from build123d import *

# Parameters (mm, degrees)
F0_R     = 5
F1_DEPTH = 15
F3_DEPTH = 12
F4_SIZE  = 0.3


with BuildPart() as f1:
    # F0 (on Top) → F1 (new body)
    with BuildSketch(Plane.XY):
        Circle(F0_R)
    extrude(amount=F1_DEPTH)

    # F2 (on face) → F3 (cut)
    with BuildSketch(Plane.XY.offset(15)):
        with BuildLine():
            Line((2.097618, 2.35), (-2.097618, 2.35))
            ThreePointArc((-2.097618, 2.35), (0, -3.15), (2.097618, 2.35))
        make_face()
    extrude(amount=-F3_DEPTH, mode=Mode.SUBTRACT)

    # F4
    f4_edges = [f1.edges().sort_by_distance(p)[0] for p in [
        (-5, 0, 0),
    ]]
    chamfer(f4_edges, length=F4_SIZE)


solid = f1.part
Model file for the job. Use its own axes, mm. A direction names the side the tool comes from. Round coordinates to 2 decimals unless told otherwise and drop trailing zeros. Loops run counter-clockwise (first coordinate to the right, second up) from the corner with the lowest first, then second, coordinate; pieces in that order, holes last.
1. Wall check: probe 1 along Y at (x, z) = (0, 10); probe 2 along Z at (x, y) = (1.5, -2); probe 3 along Y at (x, z) = (-1.75, 14). Give the ranges that are in metal, low to high.
Check values:
probe 1: y = -5 to -3.15, 2.35 to 5
probe 2: z = 0 to 3
probe 3: y = -4.68 to -2.62, 2.35 to 4.68
2. Band-saw the part on B-B, the plane y = 0. List the corners of the cut face in (x, z).
Check values:
outline: (-5, 0.3) - (-4.7, 0) - (4.7, 0) - (5, 0.3) - (5, 15) - (3.15, 15) - (3.15, 3) - (-3.15, 3) - (-3.15, 15) - (-5, 15) - close
3. Drop flat-ended pins along their axis: P1, Ø6, axis at y = -2, z = 13, coming from the -X side; P2, Ø1, axis at x = -3.5, z = 9, coming from the +Y side; P3, Ø1, axis at x = 2, y = 1, coming from the +Z side. Give the stop position or say it passes through.
Check values:
P1: stops at x = -5
P2: stops at y = 4
P3: stops at z = 3
4. Tool access for faces 1 (the flat face through (0, 0, 0)), 2 (the cylindrical face through (-0.11, -3.15, 9.08)): list every direction of +Z, -Z, +X, -X, +Y, -Y with a clear straight run to the whole face (end or side of a thin tool).
Check values:
face 1: -Z, +X, -X, +Y, -Y
face 2: +Z
5. Mould opens along Y. For faces 3 (the cylindrical face through (-1.08, -4.88, 7.55)), 4 (the flat face through (-0.1, -3.3, 15)), 5 (the flat face through (0, 0, 3)) say: +Y half, -Y half, draft (parallel to the pull), parting line (faces both ways), or undercut.
Check values:
face 3: parting line
face 4: draft
face 5: undercut
6. Band-saw the part on A-A, the plane x = 0. List the corners of the cut face in (y, z), and give its area (3 significant figures).
Check values:
outline: (-5, 0.3) - (-4.7, 0) - (4.7, 0) - (5, 0.3) - (5, 15) - (2.35, 15) - (2.35, 3) - (-3.15, 3) - (-3.15, 15) - (-5, 15) - close
area: 83.9 mm2
7. Band-saw the part on C-C, the plane z = 7.5. List the corners of the cut face in (x, y), and give its area (3 significant figures).
Check values:
outline: circle Ø10 at (0, 0); hole (-2.1, 2.35) arc R3.15 ccw (long way) to (2.1, 2.35) - close
area: 49.7 mm2
